Geometry: final body of the model. Coordinates: model frame, mm. Give positions to 0.01 mm unless a question says otherwise; leave off trailing zeros. Loops run counter-clockwise (first coordinate to the right, second up) from the corner with the lowest first, then second, coordinate; pieces in that order, holes last.
1. Material intervals for line 1 along Y through (x, z) = (0, 2.15) (3 decimals); line 2 along Z through (x, y) = (22.5, 4); line 3 along Y through (x, z) = (8, 1.5), sorted ascending.
2. Section B-B, the plane x = 11. Output: boundary loops of the cut face in (y, z).
3. Draft query along X for faces 1 (the face through (18.407, -0.088, -2.958)), 2 (the face through (11, -11, 3)), 3 (the face through (-5.51, -24.8, 1.48)). Return one class per face: +X half, -X half, draft (parallel to the pull), parting line (faces both ways), or undercut.
4. Section A-A, the plane y = -11.5. Output: boundary loops of the cut face in (x, z), then the cut area to 3 significant figures.
5. Section C-C, the plane y = -17. Output: boundary loops of the cut face in (x, z), then the cut area to 3 significant figures.
6. First-contact query: P1, Ø3, axis at x = -1.5, y = -1.5, coming from the +Z side; P2, Ø1.5, axis at y = -11.5, z = -0.5, coming from the -X side; P3, Ø5, axis at y = -10.5, z = -0.5, coming from the +X side. Flat tips, straight axial feed; report the tip coordinate or a pass-through.
from build123d import *

# Parameters (mm, degrees)
SKETCH_1_R      = 25.405
SKETCH_1_R_2    = 15.405
EXTRUDE_3_DEPTH = 3
SKETCH_4_R      = 2
EXTRUDE_4_DEPTH = 6
EXTRUDE_7_DEPTH = 0.06


# Read off the part's stored shape, not the designer's step: 填料-伸長7
with BuildPart() as part:
    # 草圖1 → 填料-伸長3 (new body)
    with BuildSketch(Plane.XY):
        Circle(SKETCH_1_R)
        Circle(SKETCH_1_R_2, mode=Mode.SUBTRACT)
    extrude(amount=EXTRUDE_3_DEPTH)

    # 草圖4 → 填料-伸長4 (add)
    with BuildSketch(Plane(origin=(0, 0, 0), x_dir=(-1, 0, 0), z_dir=(0, 0, -1))):
        with Locations(Location((20.405, 0, 0), (0, 0, 180))):
            Circle(SKETCH_4_R)
        with Locations(Location((0, 20.405, 0), (0, 0, 180))):
            Circle(SKETCH_4_R)
        with Locations(Location((-20.405, 0, 0), (0, 0, 180))):
            Circle(SKETCH_4_R)
        with Locations(Location((0, -20.405, 0), (0, 0, 180))):
            Circle(SKETCH_4_R)
    extrude(amount=EXTRUDE_4_DEPTH)

    # 填料-伸長7 outline → 填料-伸長7 (add)
    with BuildSketch(Plane(origin=(0, 0, -6), x_dir=(-1, 0, 0), z_dir=(0, 0, -1))):
        with BuildLine():
            Line((-0.435027571, 0.029718439), (-20.160544311, 1.985568742))
            ThreePointArc((-20.160544311, 1.985568742), (-22.405419947, 0.023703335), (-20.207661062, -1.990803646))
            Line((-20.207661062, -1.990803646), (-0.435027571, -0.030281561))
            ThreePointArc((-0.435027571, -0.030281561), (-0.405027571, -0.000281561), (-0.435027571, 0.029718439))
        make_face()
        with BuildLine():
            ThreePointArc((1.985568742, 20.160544311), (0.023703335, 22.405419947), (-1.990803646, 20.207661062))
            Line((-1.990803646, 20.207661062), (-0.030281561, 0.435027571))
            ThreePointArc((-0.030281561, 0.435027571), (-0.000281561, 0.405027571), (0.029718439, 0.435027571))
            Line((0.029718439, 0.435027571), (1.985568742, 20.160544311))
        make_face()
        with BuildLine():
            ThreePointArc((20.160544311, -1.985568742), (22.405419947, -0.023703335), (20.207661062, 1.990803646))
            Line((20.207661062, 1.990803646), (0.435027571, 0.030281561))
            ThreePointArc((0.435027571, 0.030281561), (0.405027571, 0.000281561), (0.435027571, -0.029718439))
            Line((0.435027571, -0.029718439), (20.160544311, -1.985568742))
        make_face()
        with BuildLine():
            ThreePointArc((-1.985568742, -20.160544311), (-0.023703335, -22.405419947), (1.990803646, -20.207661062))
            Line((1.990803646, -20.207661062), (0.030281561, -0.435027571))
            ThreePointArc((0.030281561, -0.435027571), (0.000281561, -0.405027571), (-0.029718439, -0.435027571))
            Line((-0.029718439, -0.435027571), (-1.985568742, -20.160544311))
        make_face()
    extrude(amount=EXTRUDE_7_DEPTH)


solid = part.part
Answers below:
1. line 1: y = -25.405 to -15.405, 15.405 to 25.405
1. line 2: z = 0 to 3
1. line 3: y = -24.11 to -13.16, 13.16 to 24.11
2. outline: (-22.9, 0) - (-10.78, 0) - (-10.78, 3) - (-22.9, 3) - close; (-1.08, -6.06) - (1.08, -6.06) - (1.08, -6) - (-1.08, -6) - close; (10.78, 0) - (22.9, 0) - (22.9, 3) - (10.78, 3) - close
3. face 1: undercut
3. face 2: draft
3. face 3: parting line
4. outline: (-22.65, 0) - (-10.25, 0) - (-10.25, 3) - (-22.65, 3) - close; (-1.13, -6.06) - (1.13, -6.06) - (1.13, -6) - (-1.13, -6) - close; (10.25, 0) - (22.65, 0) - (22.65, 3) - (10.25, 3) - close
4. area: 74.6 mm2
5. outline: (-18.88, 0) - (18.88, 0) - (18.88, 3) - (-18.88, 3) - close; (-1.67, -6.06) - (1.67, -6.06) - (1.67, -6) - (-1.67, -6) - close
5. area: 113 mm2
6. P1: stops at z = -6
6. P2: stops at x = -22.93
6. P3: stops at x = 24.1
